Could you check a few things on this model? Use its own coordinates, in mm. Coordinates: 2 decimals unless noted, no trailing zeros. Order: outer loops, then holes, each group sorted by start corner. A loop starts at its lowest first (then second) coordinate and runs counter-clockwise, first axis right, second up.
```python
from build123d import *

# Parameters (mm, degrees)
F1_DEPTH = 1.5
F2_R     = 4


# Not quite as in the source:
# - a feature names something its author has since deleted; it is built from what else it names


with BuildPart() as f1:
    # F0 (on Top) → F1 (new body)
    with BuildSketch(Plane.XY):
        Polygon((-160.3553390593, -14.6446609407), (-125, -50), (125, -50), (160.3553390593, -14.6446609407), (160.3553390593, 83.3553390593), (-160.3553390593, 83.3553390593), align=None)
        Polygon((-118.7867965644, -35), (-145.3553390593, -8.4314575051), (-145.3553390593, 68.3553390593), (145.3553390593, 68.3553390593), (145.3553390593, -8.4314575051), (118.7867965644, -35), align=None, mode=Mode.SUBTRACT)
        Polygon((-145.3553390593, 68.3553390593), (-145.3553390593, -8.4314575051), (-118.7867965644, -35), (118.7867965644, -35), (145.3553390593, -8.4314575051), (145.3553390593, 68.3553390593), align=None)
    extrude(amount=F1_DEPTH)

    # F2
    f2_edges = [f1.edges().sort_by_distance(p)[0] for p in [
        (160.355339, -14.644661, 0.75),
        (125, -50, 0.75),
        (160.355339, 83.355339, 0.75),
        (-125, -50, 0.75),
        (-160.355339, -14.644661, 0.75),
        (-160.355339, 83.355339, 0.75),
    ]]
    fillet(f2_edges, radius=F2_R)


solid = f1.part
```
Item 1: Suppose I cut it at B-B (x = 136). List the corners of the cut face in (y, z) for me.
Item 2: Suppose I cut it at A-A (z = 1.05). List the corners of the cut face in (x, y) for me, and give its area (3 significant figures).
Item 3: I need wall thicknesses on line 1 (X direction, y = -13.5, z = 1.2); line 2 (X direction, y = -35.5, z = 1.45); line 3 (Y direction, x = 146.5, z = 0.35). Which ranges of each line are inside material? Lowest first, please.
Geometry results:
1. outline: (-39, 0) - (83.36, 0) - (83.36, 1.5) - (-39, 1.5) - close
2. outline: (-160.36, -12.99) arc R4 ccw to (-159.18, -15.82) - (-126.17, -48.83) arc R4 ccw to (-123.34, -50) - (123.34, -50) arc R4 ccw to (126.17, -48.83) - (159.18, -15.82) arc R4 ccw to (160.36, -12.99) - (160.36, 79.36) arc R4 ccw to (156.36, 83.36) - (-156.36, 83.36) arc R4 ccw to (-160.36, 79.36) - close
2. area: 41,500 mm2
3. line 1: x = -160.32 to 160.32
3. line 2: x = -139.5 to 139.5
3. line 3: y = -28.5 to 83.36
